```python
from build123d import *

# Parameters (mm, degrees)
EXTRUDE_1_DEPTH     = 20
EXTRUDE_2_DEPTH     = 500
SKETCH_3_R          = 2.5
CUT_EXTRUDE_1_DEPTH = 250
SKETCH_4_R          = 5
CUT_EXTRUDE_2_DEPTH = 1500
CUT_EXTRUDE_3_DEPTH = 1589.363938145
SKETCH_7_R          = 15
EXTRUDE_3_DEPTH     = 60
SKETCH_8_R          = 7.5
EXTRUDE_4_DEPTH     = 60


with BuildPart() as part:
    # Эскиз1 → Бобышка-Вытянуть1 (new body)
    with BuildSketch(Plane(origin=(0, 0, 0), x_dir=(1, 0, 0), z_dir=(0, 1, 0))):
        with BuildLine():
            Line((-700, -650), (700, -650))
            ThreePointArc((700, -650), (735.355339059, -635.355339059), (750, -600))
            Line((750, -600), (750, 600))
            ThreePointArc((750, 600), (735.355339059, 635.355339059), (700, 650))
            Line((700, 650), (-700, 650))
            ThreePointArc((-700, 650), (-735.355339059, 635.355339059), (-750, 600))
            Line((-750, 600), (-750, -600))
            ThreePointArc((-750, -600), (-735.355339059, -635.355339059), (-700, -650))
        make_face()
    extrude(amount=EXTRUDE_1_DEPTH)

    # Эскиз2 → Бобышка-Вытянуть2 (add)
    with BuildSketch(Plane(origin=(0, 20, 0), x_dir=(1, 0, 0), z_dir=(0, 1, 0))):
        with BuildLine():
            Line((700, -650), (-700, -650))
            ThreePointArc((-700, -650), (-735.355339059, -635.355339059), (-750, -600))
            Line((-750, -600), (-750, 600))
            ThreePointArc((-750, 600), (-735.355339059, 635.355339059), (-700, 650))
            Line((-700, 650), (700, 650))
            ThreePointArc((700, 650), (735.355339059, 635.355339059), (750, 600))
            Line((750, 600), (750, -600))
            ThreePointArc((750, -600), (735.355339059, -635.355339059), (700, -650))
        make_face()
        with BuildLine():
            Line((665.384615385, -620), (-665.384615385, -620))
            ThreePointArc((-665.384615385, -620), (-700.739954444, -605.355339059), (-715.384615385, -570))
            Line((-715.384615385, -570), (-715.384615385, 570))
            ThreePointArc((-715.384615385, 570), (-700.739954444, 605.355339059), (-665.384615385, 620))
            Line((-665.384615385, 620), (665.384615385, 620))
            ThreePointArc((665.384615385, 620), (700.739954444, 605.355339059), (715.384615385, 570))
            Line((715.384615385, 570), (715.384615385, -570))
            ThreePointArc((715.384615385, -570), (700.739954444, -605.355339059), (665.384615385, -620))
        make_face(mode=Mode.SUBTRACT)
    extrude(amount=EXTRUDE_2_DEPTH)

    # Эскиз3 → Вырез-Вытянуть1 (cut)
    with BuildSketch(Plane.XZ):
        with Locations(Location((-650, -565, 0), (0, 0, 270))):
            Circle(SKETCH_3_R)
        with Locations(Location((-650, 565, 0), (0, 0, 270))):
            Circle(SKETCH_3_R)
        with Locations(Location((-665, 550, 0), (0, 0, 270))):
            Circle(SKETCH_3_R)
        with Locations(Location((-635, 550, 0), (0, 0, 270))):
            Circle(SKETCH_3_R)
        with Locations(Location((-650, 535, 0), (0, 0, 270))):
            Circle(SKETCH_3_R)
        with Locations(Location((665, 550, 0), (0, 0, 270))):
            Circle(SKETCH_3_R)
        with Locations(Location((650, 565, 0), (0, 0, 270))):
            Circle(SKETCH_3_R)
        with Locations(Location((635, 550, 0), (0, 0, 270))):
            Circle(SKETCH_3_R)
        with Locations(Location((650, 535, 0), (0, 0, 270))):
            Circle(SKETCH_3_R)
        with Locations(Location((650, -535, 0), (0, 0, 270))):
            Circle(SKETCH_3_R)
        with Locations(Location((635, -550, 0), (0, 0, 270))):
            Circle(SKETCH_3_R)
        with Locations(Location((665, -550, 0), (0, 0, 270))):
            Circle(SKETCH_3_R)
        with Locations(Location((650, -565, 0), (0, 0, 270))):
            Circle(SKETCH_3_R)
        with Locations(Location((-650, -535, 0), (0, 0, 270))):
            Circle(SKETCH_3_R)
        with Locations(Location((-665, -550, 0), (0, 0, 270))):
            Circle(SKETCH_3_R)
        with Locations(Location((-635, -550, 0), (0, 0, 270))):
            Circle(SKETCH_3_R)
    extrude(amount=-CUT_EXTRUDE_1_DEPTH, mode=Mode.SUBTRACT)

    # Эскиз4 → Вырез-Вытянуть2 (cut)
    with BuildSketch(Plane(origin=(0, 0, -650), x_dir=(-1, 0, 0), z_dir=(0, 0, -1))):
        with Locations((660, 260)):
            Circle(SKETCH_4_R)
    cut_extrude_2 = extrude(amount=-CUT_EXTRUDE_2_DEPTH, mode=Mode.SUBTRACT)

    # Зеркальное отражение1: Вырез-Вытянуть2 across plane
    add(cut_extrude_2.mirror(Plane.ZY), mode=Mode.SUBTRACT)

    # Эскиз6 → Вырез-Вытянуть3 (cut, through all)
    with BuildSketch(Plane(origin=(0, 0, -650), x_dir=(-1, 0, 0), z_dir=(0, 0, -1))):
        Polygon((-700, 396.571113504), (-700, 520), (-801.122226931, 520), (-801.122226931, 378.740536547), align=None)
        Polygon((-700, 396.571113504), (0, 520), (-700, 520), align=None)
        Polygon((700, 520), (0, 520), (700, 396.571113504), align=None)
        Polygon((700, 520), (700, 396.571113504), (801.122226931, 378.740536547), (801.122226931, 520), align=None)
    extrude(amount=-CUT_EXTRUDE_3_DEPTH, mode=Mode.SUBTRACT)

    # Эскиз7 → Бобышка-Вытянуть3 (add)
    with BuildSketch(Plane(origin=(0, 0, 620), x_dir=(-1, 0, 0), z_dir=(0, 0, -1))):
        with Locations((0, 420)):
            Circle(SKETCH_7_R)
    extrude_3 = extrude(amount=EXTRUDE_3_DEPTH)

    # Зеркальное отражение2: Бобышка-Вытянуть3 across plane
    add(extrude_3.mirror(Plane(origin=(0, 0, 0), x_dir=(1, 0, 0), z_dir=(0, 0, -1))))

    # Эскиз8 → Бобышка-Вытянуть4 (add)
    with BuildSketch(Plane(origin=(0, 0, 620), x_dir=(-1, 0, 0), z_dir=(0, 0, -1))):
        with Locations((0, 110)):
            Circle(SKETCH_8_R)
    extrude_4 = extrude(amount=EXTRUDE_4_DEPTH)

    # Зеркальное отражение3: Бобышка-Вытянуть4 across plane
    add(extrude_4.mirror(Plane(origin=(0, 0, 0), x_dir=(1, 0, 0), z_dir=(0, 0, -1))))


solid = part.part
```
Verification items for the finished model (mm, model axes). A direction names the side the tool comes from. Give positions to 0.01 mm unless a question says otherwise; leave off trailing zeros. Order: outer loops, then holes, each group sorted by start corner. A loop starts at its lowest first (then second) coordinate and runs counter-clockwise, first axis right, second up. Notation, with made-up numbers: (31.25, 4.25) -> (61.25, 4.25) arc R23 cw to (61.25, 17.25) -> close; hole circle Ø11 at (-30.5, -35). An arc over 180 degrees is marked (long way). One line per item, written item: value.
(1) Sectioned sample at B-B on z = -17. Record the cut outline in (x, y).
Final values:
outline: (-750, 0) -> (750, 0) -> (750, 387.75) -> (715.38, 393.86) -> (715.38, 20) -> (-715.38, 20) -> (-715.38, 393.86) -> (-750, 387.75) -> close
(2) Gauge pin test, flat end, axial feed: pin 1 (8 mm diameter, centred on x = 665, z = 550, fed in from +Y). Record the tip position at first contact, or that the pin passes through.
Final values:
pin 1: y = 20
(3) Draft check along Z on faces 1 (the face through (700.35, 208.66, -605.74)), 2 (the face through (10, 256, 650)), 3 (the face through (-10, 0, -9)), 4 (the face through (-10, 256, -650)). Enter one of: pulls with the +Z half, pulls with the -Z half, needs draft (parallel to the pull), parting line crosses it, or undercut.
Final values:
face 1: undercut
face 2: pulls with the +Z half
face 3: needs draft
face 4: pulls with the -Z half
(4) Tool access check on faces 5 (the face through (701.13, 208.66, 604.96)), 6 (the face through (-735.742, 195.51, -634.964)). Record the directions out of +Z, -Z, +X, -X, +Y, -Y that give a thin tool (end or side, any length) a straight path to the whole face; none if there is none.
Final values:
face 5: +Y
face 6: -Z, -X, +Y, -Y
(5) Scan lines: line 1 along Z through (x, y) = (665, 10.75); line 2 along X through (y, z) = (15, 550); line 3 along Z through (x, y) = (341, 164.5). Record each from-to range of solid material in increasing order. Write a range as [from, to].
Final values:
line 1: [-650, -552.5], [-547.5, 547.5], [552.5, 650]
line 2: [-750, -667.5], [-662.5, -637.5], [-632.5, 632.5], [637.5, 662.5], [667.5, 750]
line 3: [-650, -620], [620, 650]
(6) Sectioned sample at A-A on y = 361.5. Record the cut outline in (x, z).
Final values:
outline: (-750, -600) arc R50 ccw to (-700, -650) -> (700, -650) arc R50 ccw to (750, -600) -> (750, 600) arc R50 ccw to (700, 650) -> (-700, 650) arc R50 ccw to (-750, 600) -> close; hole (-715.38, -570) arc R50 ccw to (-665.38, -620) -> (665.38, -620) arc R50 ccw to (715.38, -570) -> (715.38, 570) arc R50 ccw to (665.38, 620) -> (-665.38, 620) arc R50 ccw to (-715.38, 570) -> close
(7) Sectioned sample at C-C on x = -581.5. Record the cut outline in (y, z).
Final values:
outline: (0, -650) -> (417.47, -650) -> (417.47, -620) -> (20, -620) -> (20, 620) -> (417.47, 620) -> (417.47, 650) -> (0, 650) -> close
